For this review, take the finished solid that the model builds, in its own axes (mm). Give positions to 0.01 mm unless a question says otherwise; leave off trailing zeros. Order: outer loops, then holes, each group sorted by start corner. A loop starts at its lowest first (then second) coordinate and runs counter-clockwise, first axis right, second up.
from build123d import *

# Parameters (mm, degrees)
SKETCH_1_W          = 102
SKETCH_1_H          = 102
SKETCH_1_R          = 1.5
SKETCH_1_R_2        = 1
EXTRUDE_1_DEPTH     = 2
SKETCH_2_W          = 92
SKETCH_2_H          = 68
CUT_EXTRUDE_1_DEPTH = 10
SKETCH_3_W          = 68
SKETCH_3_H          = 92
CUT_EXTRUDE_2_DEPTH = 10
FILLET_1_R          = 4
CUT_EXTRUDE_3_DEPTH = 10
FILLET_2_R          = 1


with BuildPart() as part:
    # 草图1 → 凸台-拉伸1 (new body)
    with BuildSketch(Plane(origin=(0, 0, 0), x_dir=(1, 0, 0), z_dir=(0, 1, 0))):
        with Locations((-50.486691813, 4.007835052)):
            Rectangle(SKETCH_1_W, SKETCH_1_H)
        with Locations(Location((-95.686691813, -43.492164948, 0), (0, 0, 270))):
            Circle(SKETCH_1_R, mode=Mode.SUBTRACT)
        with Locations(Location((-95.686691813, 51.507835052, 0), (0, 0, 270))):
            Circle(SKETCH_1_R, mode=Mode.SUBTRACT)
        with Locations(Location((-5.286691813, -43.492164948, 0), (0, 0, 270))):
            Circle(SKETCH_1_R, mode=Mode.SUBTRACT)
        with Locations(Location((-5.286691813, 51.507835052, 0), (0, 0, 270))):
            Circle(SKETCH_1_R, mode=Mode.SUBTRACT)
        with Locations(Location((-90.486691813, -35.992164948, 0), (0, 0, 270))):
            Circle(SKETCH_1_R_2, mode=Mode.SUBTRACT)
        with Locations(Location((-90.486691813, 44.007835052, 0), (0, 0, 270))):
            Circle(SKETCH_1_R_2, mode=Mode.SUBTRACT)
        with Locations(Location((-10.486691813, -35.992164948, 0), (0, 0, 270))):
            Circle(SKETCH_1_R_2, mode=Mode.SUBTRACT)
        with Locations(Location((-10.486691813, 44.007835052, 0), (0, 0, 270))):
            Circle(SKETCH_1_R_2, mode=Mode.SUBTRACT)
    extrude(amount=EXTRUDE_1_DEPTH)

    # 草图2 → 切除-拉伸1 (cut)
    with BuildSketch(Plane(origin=(0, 2, 0), x_dir=(1, 0, 0), z_dir=(0, 1, 0))):
        with Locations((-50.486691813, 4.007835052)):
            Rectangle(SKETCH_2_W, SKETCH_2_H)
    extrude(amount=-CUT_EXTRUDE_1_DEPTH, mode=Mode.SUBTRACT)

    # 草图3 → 切除-拉伸2 (cut)
    with BuildSketch(Plane(origin=(0, 2, 0), x_dir=(1, 0, 0), z_dir=(0, 1, 0))):
        with Locations((-50.486691813, 4.007835052)):
            Rectangle(SKETCH_3_W, SKETCH_3_H)
    extrude(amount=-CUT_EXTRUDE_2_DEPTH, mode=Mode.SUBTRACT)

    # 圆角1
    fillet_1_edges = [part.edges().sort_by_distance(p)[0] for p in [
        (0.513308187, 1, -55.007835052),
        (0.513308187, 1, 46.992164948),
        (-101.486691813, 1, 46.992164948),
        (-101.486691813, 1, -55.007835052),
    ]]
    fillet(fillet_1_edges, radius=FILLET_1_R)

    # 草图4 → 切除-拉伸3 (cut)
    with BuildSketch(Plane(origin=(0, 2, 0), x_dir=(1, 0, 0), z_dir=(0, 1, 0))):
        with BuildLine():
            Line((-89.047351985, 40.44717488), (-92.58288589, 43.982708786))
            ThreePointArc((-92.58288589, 43.982708786), (-92.58288589, 46.104029129), (-90.461565547, 46.104029129))
            Line((-90.461565547, 46.104029129), (-86.926031641, 42.568495223))
            ThreePointArc((-86.926031641, 42.568495223), (-86.926031641, 40.44717488), (-89.047351985, 40.44717488))
        make_face()
        with BuildLine():
            Line((-14.047351985, 42.568495223), (-10.511818079, 46.104029129))
            ThreePointArc((-10.511818079, 46.104029129), (-8.390497735, 46.104029129), (-8.390497735, 43.982708786))
            Line((-8.390497735, 43.982708786), (-11.926031641, 40.44717488))
            ThreePointArc((-11.926031641, 40.44717488), (-14.047351985, 40.44717488), (-14.047351985, 42.568495223))
        make_face()
        with BuildLine():
            Line((-11.926031641, -32.431504777), (-8.390497735, -35.967038683))
            ThreePointArc((-8.390497735, -35.967038683), (-8.390497735, -38.088359026), (-10.511818079, -38.088359026))
            Line((-10.511818079, -38.088359026), (-14.047351985, -34.55282512))
            ThreePointArc((-14.047351985, -34.55282512), (-14.047351985, -32.431504777), (-11.926031641, -32.431504777))
        make_face()
        with BuildLine():
            Line((-86.926031641, -34.55282512), (-90.461565547, -38.088359026))
            ThreePointArc((-90.461565547, -38.088359026), (-92.58288589, -38.088359026), (-92.58288589, -35.967038683))
            Line((-92.58288589, -35.967038683), (-89.047351985, -32.431504777))
            ThreePointArc((-89.047351985, -32.431504777), (-86.926031641, -32.431504777), (-86.926031641, -34.55282512))
        make_face()
    extrude(amount=-CUT_EXTRUDE_3_DEPTH, mode=Mode.SUBTRACT)

    # 圆角2
    fillet_2_edges = [part.edges().sort_by_distance(p)[0] for p in [
        (-96.486691813, 1, 29.992164948),
        (-96.486691813, 1, -38.007835052),
        (-4.486691813, 1, -38.007835052),
        (-4.486691813, 1, 29.992164948),
        (-16.486691813, 1, 29.992164948),
        (-84.486691813, 1, 29.992164948),
        (-84.486691813, 1, -38.007835052),
        (-16.486691813, 1, -50.007835052),
        (-16.486691813, 1, -38.007835052),
        (-84.486691813, 1, 41.992164948),
        (-84.486691813, 1, -50.007835052),
        (-16.486691813, 1, 41.992164948),
    ]]
    fillet(fillet_2_edges, radius=FILLET_2_R)


solid = part.part
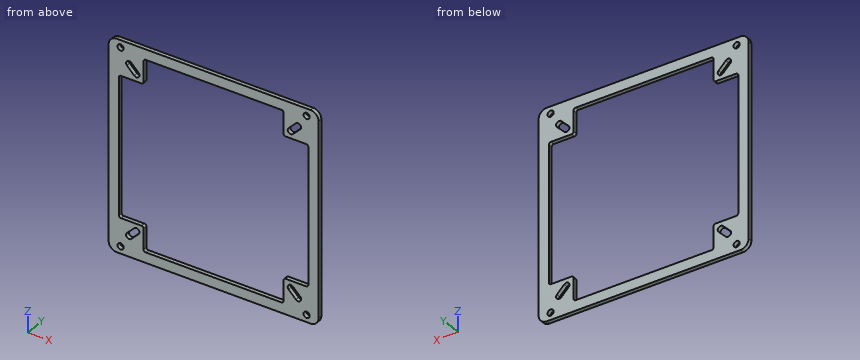
1) To check wall thickness, follow line 1 (Z direction, x = -5.5, y = 0.1); line 2 (X direction, y = 0.1, z = 12.5); line 3 (Z direction, x = -83.5, y = 1.7). State the ranges of each line that lie inside material, in increasing order.
Answer sheet:
line 1: z = -55.01 to -52.99, -50.02 to -38.01, 29.99 to 42.01, 44.98 to 46.99
line 2: x = -101.49 to -96.49, -4.49 to 0.51
line 3: z = -55.01 to -50.01, 41.99 to 46.99
2) Clearance check with a flat-ended pin moving along its axis: pin 1 (4 mm diameter, centred on x = -95.69, z = 43.49, fed in from -Y). State where the tip first meets the part, or that it passes through.
Answer sheet:
pin 1: stops at y = 0
3) We need section A-A on x = -45. Give the boundary of the cut face in (y, z).
Answer sheet:
outline: (0, -55.01) - (2, -55.01) - (2, -50.01) - (0, -50.01) - close; (0, 41.99) - (2, 41.99) - (2, 46.99) - (0, 46.99) - close
4) We need section C-C on y = 0.55. Count the separate pieces of the cut face and the enclosed holes in it, then the cut area to 3 significant figures.
Answer sheet:
separate pieces: 1
enclosed holes: 9
area: 2,390 mm2
5) We need section B-B on z = 17.5. Give the boundary of the cut face in (x, y), then the cut area to 3 significant figures.
Answer sheet:
outline: (-101.49, 0) - (-96.49, 0) - (-96.49, 2) - (-101.49, 2) - close; (-4.49, 0) - (0.51, 0) - (0.51, 2) - (-4.49, 2) - close
area: 20.0 mm2
